from build123d import *

# Parameters (mm, degrees)
SKETCH_1_W      = 100
SKETCH_1_H      = 100
EXTRUDE_1_DEPTH = 50
EXTRUDE_2_DEPTH = 5


with BuildPart() as part:
    # Sketch 1 → Extrude 1 (new, symmetric)
    with BuildSketch(Plane.XY):
        Rectangle(SKETCH_1_W, SKETCH_1_H)
    extrude(amount=EXTRUDE_1_DEPTH, both=True)

    # Sketch 1_3 → Extrude 2 (add, symmetric)
    with BuildSketch(Plane.XY):
        Polygon((-90.014973854, -40), (-50, -15), (-50, 15), (-90, 40), (-250, 40), (-250, -40), align=None)
        Polygon((50, 15), (50, -15), (90, -40), (250, -40), (250, 40), (90, 40), align=None)
    extrude(amount=EXTRUDE_2_DEPTH, both=True)


solid = part.part
Work out the finished part from the listing and answer in its coordinate system (mm). A direction names the side the tool comes from. Give positions to 0.01 mm unless a question says otherwise; leave off trailing zeros. Loops run counter-clockwise (first coordinate to the right, second up) from the corner with the lowest first, then second, coordinate; pieces in that order, holes last. Notation, with made-up numbers: (53.25, 70) - (101.25, 70) arc R24 cw to (101.25, 91) - close; hole circle Ø11 at (-1.75, 77). An arc over 180 degrees is marked (long way). Answer in a Markdown table with one row per item. Add a question column.
Q1. The part is cut by section C-C (x = -175). Determine the outline of the cut face in (y, z).
Q2. Each of these flat-tipped pins is pushed along its axis until it touches: P1, Ø3, axis at x = -189, z = 0, coming from the -Y side; P2, Ø8, axis at x = 166.5, z = -2, coming from the +Y side; P3, Ø24, axis at x = 178, y = -16, coming from the -Z side. Where does it stop, or does it pass through?
Q3. Determine the mould class of faces 5 (the flat face through (169, -40, 0)), 6 (the flat face through (250, -1, 0)), 7 (the flat face through (69.72, -27.325, 0.07)) for opening direction X: released by +X, released by -X, zero draft, split by the parting line, or undercut.
Q4. The part is cut by section A-A (y = 35.5). Determine the outline of the cut face in (x, z), and give its area (3 significant figures).
Q5. A tool of negligible diameter and unlimited length cuts with its end or side. For faces 1 (the flat face through (-151, 1, 5)), 2 (the flat face through (-171, -40, 0)), 3 (the flat face through (70.28, 27.675, 0.07)), 4 (the flat face through (171, 40, 0)), from which of +Z, -Z, +X, -X, +Y, -Y can it reach the whole face along a straight path? Write none if from no direction.
Q6. Consider line 1 along X through (y, z) = (27, 0); line 2 along X through (y, z) = (-17.5, 44.5); line 3 along Z through (x, y) = (191.5, -18). Determine where each line is inside the solid, lowest interval first.
Q7. The part is cut by section D-D (z = -36). Determine the outline of the cut face in (x, y), and give its area (3 significant figures).
Q8. The part is cut by section B-B (y = -1.5). Determine the outline of the cut face in (x, z), and give its area (3 significant figures).
Solution:
| question | item | result |
|---|---|---|
| 1 | outline | (-40, -5) - (40, -5) - (40, 5) - (-40, 5) - close |
| 2 | P1 | stops at y = -40 |
| 2 | P2 | stops at y = 40 |
| 2 | P3 | stops at z = -5 |
| 3 | face 5 | zero draft |
| 3 | face 6 | released by +X |
| 3 | face 7 | undercut |
| 4 | outline | (-250, -5) - (-82.8, -5) - (-82.8, 5) - (-250, 5) - close; (-50, -50) - (50, -50) - (50, 50) - (-50, 50) - close; (82.8, -5) - (250, -5) - (250, 5) - (82.8, 5) - close |
| 4 | area | 13,300 mm² |
| 5 | face 1 | +Z, -X, +Y, -Y |
| 5 | face 2 | +Z, -Z, -X, -Y |
| 5 | face 3 | +Z, -Z, +Y |
| 5 | face 4 | +Z, -Z, +X, +Y |
| 6 | line 1 | x = -250 to -69.2, -50 to 50, 69.2 to 250 |
| 6 | line 2 | x = -50 to 50 |
| 6 | line 3 | z = -5 to 5 |
| 7 | outline | (-50, -50) - (50, -50) - (50, 50) - (-50, 50) - close |
| 7 | area | 10,000 mm² |
| 8 | outline | (-250, -5) - (-50, -5) - (-50, -50) - (50, -50) - (50, -5) - (250, -5) - (250, 5) - (50, 5) - (50, 50) - (-50, 50) - (-50, 5) - (-250, 5) - close |
| 8 | area | 14,000 mm² |
